```python
from build123d import *

# Parameters (mm, degrees)
F0_W      = 76.2
F0_H      = 73.66
F0_R      = 1.905
F1_DEPTH  = 3.81
F2_SIZE   = 1.27
F3_SIZE   = 2.54
F5_DEPTH  = 73.66
F6_R      = 7.94385
F6_R_2    = 0.79375
F7_DEPTH  = 49.3924086659
F9_W      = 45.7835
F9_H      = 20.9296
F9_W_2    = 45.2755
F9_H_2    = 20.4216
F9_R      = 0.79375
F10_DEPTH = 25.4
F12_DEPTH = 76.201
F13_R     = 2.54


with BuildPart() as f1:
    # F0 (on Top) → F1 (new body)
    with BuildSketch(Plane.XY):
        with Locations((-41.9906750321, 50.2695810336)):
            Rectangle(F0_W, F0_H)
        with Locations((-76.2806750321, 17.2495810336)):
            Circle(F0_R, mode=Mode.SUBTRACT)
        with Locations((-6.4306750321, 17.2495810336)):
            Circle(F0_R, mode=Mode.SUBTRACT)
        with Locations((-76.2806750321, 83.2895810336)):
            Circle(F0_R, mode=Mode.SUBTRACT)
        with Locations((-6.4306750321, 83.2895810336)):
            Circle(F0_R, mode=Mode.SUBTRACT)
    extrude(amount=F1_DEPTH)

    # F2
    f2_edges = [f1.edges().sort_by_distance(p)[0] for p in [
        (-3.890675, 13.439581, 1.905),
        (-3.890675, 87.099581, 1.905),
    ]]
    chamfer(f2_edges, length=F2_SIZE)

    # F3
    f3_edges = [f1.edges().sort_by_distance(p)[0] for p in [
        (-80.090675, 13.439581, 1.905),
        (-80.090675, 87.099581, 1.905),
    ]]
    chamfer(f3_edges, length=F3_SIZE)

    # F4 (on face) → F5 (join, through all)
    with BuildSketch(Plane.XZ.offset(-13.4395810336)):
        Polygon((-51.97016279, 21.7705122421), (-69.9306750321, 3.81), (-34.0096505479, 3.81), align=None)
    extrude(amount=-F5_DEPTH)

    # F6 (on face) → F7 (cut, through all)
    with BuildSketch(Plane(origin=(-36.8703375161, 0, 36.8703375161), x_dir=(0, -1, 0), z_dir=(-0.7071067812, 0, 0.7071067812))):
        with Locations((-62.9886310336, -34.2575776919)):
            Circle(F6_R)
        with Locations((-37.5505310336, -34.2575776919)):
            Circle(F6_R)
        with Locations((-29.1558310336, -25.5707776919)):
            Circle(F6_R_2)
        with Locations((-29.1558310336, -42.9443776919)):
            Circle(F6_R_2)
        with Locations((-71.3833310336, -42.9443776919)):
            Circle(F6_R_2)
        with Locations((-71.3833310336, -25.5707776919)):
            Circle(F6_R_2)
    extrude(amount=-F7_DEPTH, mode=Mode.SUBTRACT)

    # F9 (on offset) → F10 (cut)
    with BuildSketch(Plane(origin=(-28.2492916398, 0, 28.2492916398), x_dir=(0, -1, 0), z_dir=(-0.7071067812, 0, 0.7071067812))):
        with Locations((-50.2695810336, -34.2575776919)):
            Rectangle(F9_W, F9_H)
        with Locations((-50.2695810336, -34.2575776919)):
            Rectangle(F9_W_2, F9_H_2, mode=Mode.SUBTRACT)
        with Locations((-50.2695810336, -34.2575776919)):
            Rectangle(F9_W_2, F9_H_2)
        with Locations((-71.3833310336, -42.9443776919)):
            Circle(F9_R, mode=Mode.SUBTRACT)
        with Locations((-29.1558310336, -42.9443776919)):
            Circle(F9_R, mode=Mode.SUBTRACT)
        with Locations((-71.3833310336, -25.5707776919)):
            Circle(F9_R, mode=Mode.SUBTRACT)
        with Locations((-29.1558310336, -25.5707776919)):
            Circle(F9_R, mode=Mode.SUBTRACT)
        with Locations((-29.1558310336, -25.5707776919)):
            Circle(F9_R)
        with Locations((-29.1558310336, -42.9443776919)):
            Circle(F9_R)
        with Locations((-71.3833310336, -42.9443776919)):
            Circle(F9_R)
        with Locations((-71.3833310336, -25.5707776919)):
            Circle(F9_R)
    extrude(amount=-F10_DEPTH, mode=Mode.SUBTRACT)

    # F11 (on face) → F12 (cut, through all)
    with BuildSketch(Plane(origin=(-80.0906750321, 0, 0), x_dir=(0, -1, 0), z_dir=(-1, 0, 0))):
        Polygon((-84.5595810336, 3.81), (-75.7013310336, 3.81), (-75.7013310336, 27.0840693265), (-94.177685678, 27.0840693265), (-93.6518386006, 3.81), align=None)
        Polygon((-24.8378310336, 27.0840693265), (-24.8378310336, 3.81), (-15.9795810336, 3.81), (-6.8873234665, 3.81), (-6.3614763892, 27.0840693265), align=None)
    extrude(amount=-F12_DEPTH, mode=Mode.SUBTRACT)

    # F13
    f13_edges = [f1.edges().sort_by_distance(p)[0] for p in [
        (-51.970163, 50.269581, 21.770512),
    ]]
    fillet(f13_edges, radius=F13_R)


solid = f1.part
```
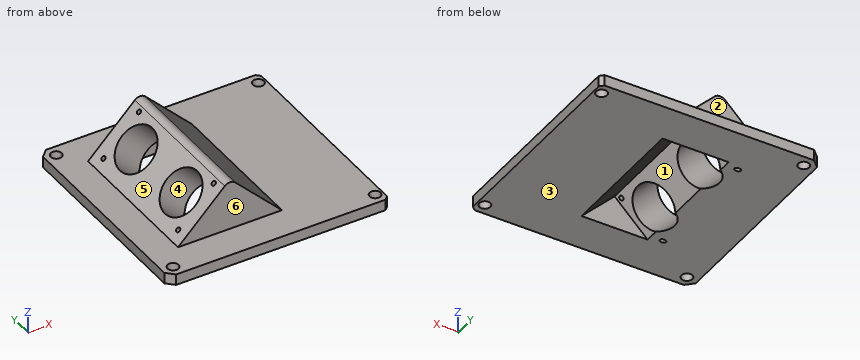
Check sheet for the modelled part. Datum: model origin and axes. Units: mm. Face numbers are marked on the shaded views. A direction names the side the tool comes from. Give positions to 0.01 mm unless a question says otherwise; leave off trailing zeros. Order: outer loops, then holes, each group sorted by start corner. A loop starts at its lowest first (then second) coordinate and runs counter-clockwise, first axis right, second up. Notation, with made-up numbers: (72, -2) -> (94, -2) arc R22 ccw to (94, 4) -> close; hole circle Ø7 at (-28, 24.5). An arc over 180 degrees is marked (long way). Use CSV: the item, a comma, the result in double quotes. Start each with the question number.
1) Sectioned sample at A-A, the plane y = 63. Record the boundary of the cut face in (x, z).
2) Material ranges on line 1 (X direction, y = 19, z = 3.25); line 2 (Y direction, x = -46, z = 14.5); line 3 (Y direction, x = -56, z = 10.5), recorded low to high. Write a range as from..to.
3) Set-up check for the marked faces 1, 2 and 3: record each of +Z, -Z, +X, -X, +Y, -Y from which the full face is reachable in a straight line by a thin tool's end or side.
4) Sectioned sample at D-D, the plane z = 1.5. Give the number of separate pieces and of enclosed holes in the cut face, plus the area to 3 significant figures.
5) Mould release check, pull along X, two halves, no side actions. Record for the marked faces 4, 5 and 6: released by +X, released by -X, zero draft, split by the parting line, or undercut.
6) Sectioned sample at B-B, the plane x = -36. Record the boundary of the cut face in (y, z), plus the area to 3 significant figures.
7) Go/stop test with flat-tipped pins: P1, Ø12, axis at x = -23, y = 23.5, coming from the +Z side; P2, Ø8.5, axis at x = -45.5, z = 12.5, coming from the -Y side; P3, Ø6, axis at x = -35, z = 7, coming from the +Y side. Record where each tip stops, or that it passes through.
8) Sectioned sample at C-C, the plane y = 49. Record the boundary of the cut face in (x, z).
Recorded:
1,outline,"(-80.09, 0) -> (-59.68, 0) -> (-66.71, 7.03) -> (-69.93, 3.81) -> (-80.09, 3.81) -> close; (-55.48, 18.26) -> (-46.86, 9.64) -> (-45.07, 11.43) -> (-33.65, 0) -> (-3.89, 0) -> (-3.89, 3.81) -> (-34.01, 3.81) -> (-50.17, 19.97) arc R2.54 ccw to (-53.77, 19.97) -> close"
2,line 1,"-80.09..-77.03, -75.53..-7.18, -5.68..-3.89"
2,line 2,"24.84..75.7"
2,line 3,"24.84..29.88, 45.22..55.32, 70.65..75.7"
3,face 1,"-Z"
3,face 2,"+Z, +X, -X, +Y"
3,face 3,"-Z, +X, -X, +Y, -Y"
4,separate pieces,"1"
4,enclosed holes,"7"
4,area,"4,520 mm2"
5,face 4,"undercut"
5,face 5,"released by -X"
5,face 6,"zero draft"
6,outline,"(13.44, 0) -> (27.38, 0) -> (27.38, 2.35) -> (73.16, 2.35) -> (73.16, 0) -> (87.1, 0) -> (87.1, 3.81) -> (75.7, 3.81) -> (75.7, 5.8) -> (24.84, 5.8) -> (24.84, 3.81) -> (13.44, 3.81) -> close"
6,area,"274 mm2"
7,P1,"z = 3.81"
7,P2,"y = 24.84"
7,P3,"y = 75.7"
8,outline,"(-80.09, 0) -> (-56.5, 0) -> (-45.07, 11.43) -> (-33.65, 0) -> (-3.89, 0) -> (-3.89, 3.81) -> (-34.01, 3.81) -> (-50.17, 19.97) arc R2.54 ccw to (-53.77, 19.97) -> (-69.93, 3.81) -> (-80.09, 3.81) -> close"
